Geometry: see drawing. Coordinates: mm, zero at the bounding-box minimum. Give positions to 0.01 mm unless a question says otherwise; leave off trailing zeros. Write each loop counter-clockwise with the first axis right and the second up, starting at its lowest first coordinate (ties: lowest second). Pieces come first, ordered by that corner, then holes. Notation, with made-up numbers: (84.5, 10.5) -> (102.5, 10.5) arc R17 cw to (102.5, 24.5) -> close; hole circle Ø6 at (40, -11.75). An arc over 180 degrees is marked (long way). Use CSV: the item, a comma, the result in double quotes. Start each with the question number.
1) Material intervals for line 1 (Y direction, x = 13.5, z = 2.45); line 2 (Y direction, x = 22, z = 1.95); line 3 (Y direction, x = 24.5, z = 2), sorted ascending. Write a range as [from, to].
2) Section A-A (x = 21.5). Output: boundary loops of the cut face in (y, z).
3) Section B-B (y = 16). Output: boundary loops of the cut face in (x, z), plus the area to 3 significant figures.
4) Section D-D (x = 13.5). Output: boundary loops of the cut face in (y, z), plus the area to 3 significant figures.
5) Section C-C (z = 3.05). Output: boundary loops of the cut face in (x, y), plus the area to 3 significant figures.
6) Draft query along Y for the marked faces 1, 2 and 3. Return one class per face: pulls with the +Y half, pulls with the -Y half, needs draft (parallel to the pull), parting line crosses it, or undercut.
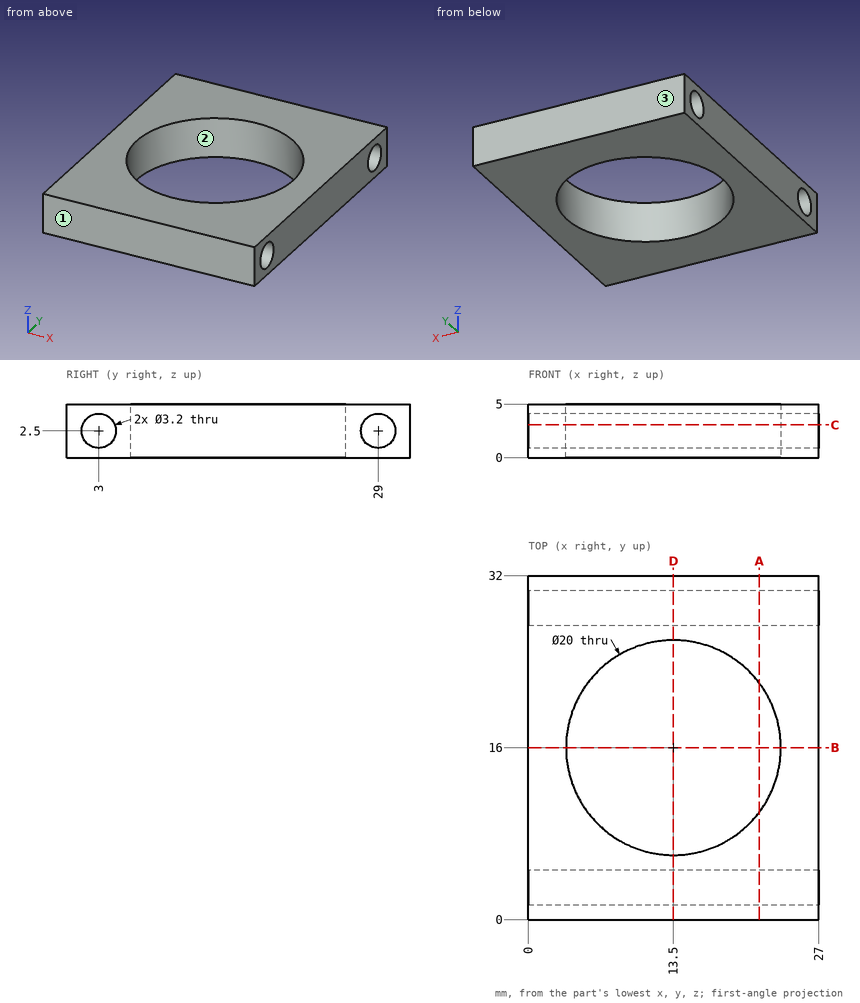
Answers follow:
1,line 1,"y = [0, 1.4], [4.6, 6], [26, 27.4], [30.6, 32]"
1,line 2,"y = [0, 1.5], [4.5, 10.73], [21.27, 27.5], [30.5, 32]"
1,line 3,"y = [0, 1.48], [4.52, 27.48], [30.52, 32]"
2,outline,"(0, 0) -> (10, 0) -> (10, 5) -> (0, 5) -> close; (22, 0) -> (32, 0) -> (32, 5) -> (22, 5) -> close; hole circle Ø3.2 at (3, 2.5); hole circle Ø3.2 at (29, 2.5)"
3,outline,"(0, 0) -> (3.5, 0) -> (3.5, 5) -> (0, 5) -> close; (23.5, 0) -> (27, 0) -> (27, 5) -> (23.5, 5) -> close"
3,area,"35.0 mm^2"
4,outline,"(0, 0) -> (6, 0) -> (6, 5) -> (0, 5) -> close; (26, 0) -> (32, 0) -> (32, 5) -> (26, 5) -> close; hole circle Ø3.2 at (3, 2.5); hole circle Ø3.2 at (29, 2.5)"
4,area,"43.9 mm^2"
5,outline,"(0, 0) -> (27, 0) -> (27, 1.5) -> (0, 1.5) -> close; (0, 4.5) -> (27, 4.5) -> (27, 27.5) -> (0, 27.5) -> close; (0, 30.5) -> (27, 30.5) -> (27, 32) -> (0, 32) -> close; hole circle Ø20 at (13.5, 16)"
5,area,"388 mm^2"
6,face 1,"pulls with the -Y half"
6,face 2,"undercut"
6,face 3,"pulls with the +Y half"
